For this review, take the finished solid that the model builds, in its own axes (mm). Coordinates: 2 decimals unless noted, no trailing zeros. Write each loop counter-clockwise with the first axis right and the second up, starting at its lowest first coordinate (ties: lowest second). Pieces come first, ordered by that corner, then holes. Notation, with made-up numbers: (25, 14.5) - (33, 14.5) arc R26 ccw to (33, 43.5) - close; hole circle Ø5 at (76, 7.25). An arc over 180 degrees is marked (long way). Write each question's results on one line, items separated by ' | '.
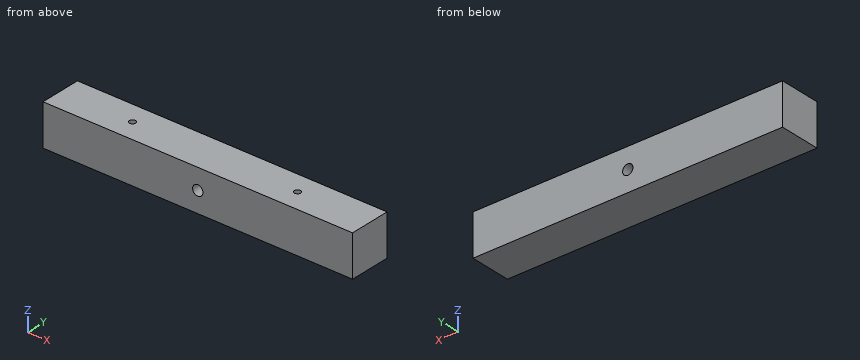
from build123d import *

# Parameters (mm, degrees)
F0_W     = 150
F0_H     = 20
F1_DEPTH = 20
F2_R     = 1.5
F3_DEPTH = 10
F4_R     = 2.5
F5_DEPTH = 25


with BuildPart() as f1:
    # F0 (on Top) → F1 (new body)
    with BuildSketch(Plane.XY):
        Rectangle(F0_W, F0_H)
    extrude(amount=F1_DEPTH)

    # F2 (on face) → F3 (cut)
    with BuildSketch(Plane.XY.offset(20)):
        with Locations((40, 0)):
            Circle(F2_R)
        with Locations((-40, 0)):
            Circle(F2_R)
    extrude(amount=-F3_DEPTH, mode=Mode.SUBTRACT)

    # F4 (on face) → F5 (cut)
    with BuildSketch(Plane.XZ.offset(10)):
        with Locations((0, 10)):
            Circle(F4_R)
    extrude(amount=-F5_DEPTH, mode=Mode.SUBTRACT)


solid = f1.part
Q1. Take a section at A-A on y = 0. State the section outline as (x, z) points, plus the area to 3 significant figures.
Results found:
outline: (-75, 0) - (75, 0) - (75, 20) - (41.5, 20) - (41.5, 10) - (38.5, 10) - (38.5, 20) - (-38.5, 20) - (-38.5, 10) - (-41.5, 10) - (-41.5, 20) - (-75, 20) - close; hole circle Ø5 at (0, 10) | area: 2,920 mm2
Q2. Take a section at B-B on x = 0. State the section outline as (y, z) points, plus the area to 3 significant figures.
Results found:
outline: (-10, 0) - (10, 0) - (10, 7.5) - (-10, 7.5) - close; (-10, 12.5) - (10, 12.5) - (10, 20) - (-10, 20) - close | area: 300 mm2
Q3. For pin 1 (0.9 mm diameter, centred on x = -40, y = 0, fed in from +Z), flat-tipped, find the tip position at first contact; note if it passes through.
Results found:
pin 1: z = 10
Q4. Wall thickness on line 1 along Y through (x, z) = (-40, 14.75); line 2 along Z through (x, y) = (0, 0.25); line 3 along X through (y, z) = (1, 18.5): over which ranges is each line inside the solid? List them lowest first. Write a range as from..to.
Results found:
line 1: -10..-1.5, 1.5..10 | line 2: 0..7.5, 12.5..20 | line 3: -75..-41.12, -38.88..38.88, 41.12..75
Q5. Take a section at C-C on x = 40. State the section outline as (y, z) points.
Results found:
outline: (-10, 0) - (10, 0) - (10, 20) - (1.5, 20) - (1.5, 10) - (-1.5, 10) - (-1.5, 20) - (-10, 20) - close
